Drawing for the job (mm, zero at the part's lowest x, y, z). Coordinates: 2 decimals unless noted, no trailing zeros. Loops run counter-clockwise (first coordinate to the right, second up) from the corner with the lowest first, then second, coordinate; pieces in that order, holes last. Notation, with made-up numbers: (59, 35) - (88, 35) arc R29 ccw to (88, 62) - close; hole circle Ø6 at (34.25, 50). An arc over 180 degrees is marked (long way). One line per item, written item: value.
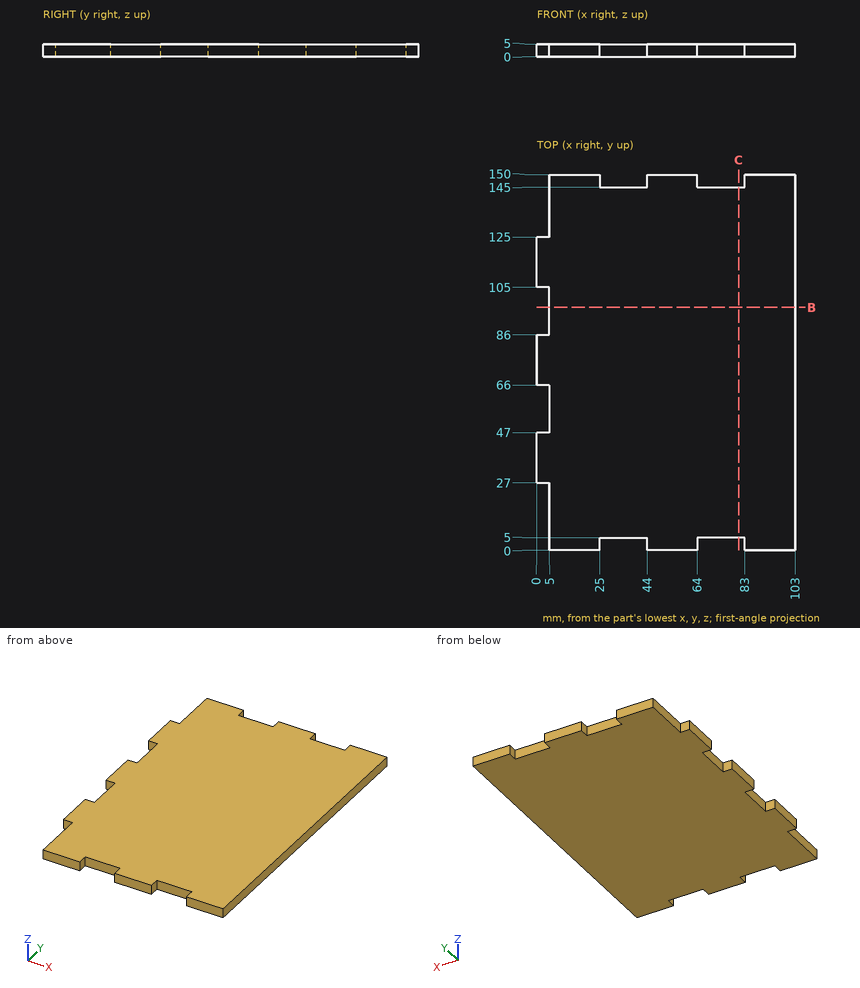
Item 1: Cut at C-C, the plane x = 80.5. Write the cut outline in (y, z), then the cut area to 3 significant figures.
Check result:
outline: (5, 0) - (145, 0) - (145, 5) - (5, 5) - close
area: 700 mm^2
Item 2: Probe probe 1 along X at (y, z) = (132, 4.15); probe 2 along Y at (x, z) = (79, 2.8). List the from-to ranges inside material, lowest first. Write a range as from..to.
Check result:
probe 1: x = 5..103
probe 2: y = 5..145
Item 3: Cut at B-B, the plane y = 97. Write the cut outline in (x, z).
Check result:
outline: (5, 0) - (103, 0) - (103, 5) - (5, 5) - close
Item 4: Drop flat-ended pins along their axis: P1, Ø2.5, axis at x = 76, z = 2.5, coming from the +Y side; P2, Ø2.5, axis at x = 72.5, z = 1.5, coming from the -Y side; P3, Ø2.5, axis at x = 3, z = 2, coming from the -Y side. Give the stop position or say it passes through.
Check result:
P1: stops at y = 145
P2: stops at y = 5
P3: stops at y = 27
